Model file for the job. Use its own axes, mm. A direction names the side the tool comes from. Round coordinates to 2 decimals unless told otherwise and drop trailing zeros. Loops run counter-clockwise (first coordinate to the right, second up) from the corner with the lowest first, then second, coordinate; pieces in that order, holes last.
from build123d import *

# Parameters (mm, degrees)
BOSS_EXTRUDE1_DEPTH = 6


with BuildPart() as part:
    # Sketch1 → Boss-Extrude1 (new body)
    with BuildSketch(Plane.XY):
        Polygon((24.866162055, -35.317756725), (12.866162055, -35.317756725), (12.866162055, -26.332846246), (-17.133837945, -26.332846246), (-17.133837945, -35.317756725), (-29.133837945, -35.317756725), (-29.133837945, -53.317756725), (-17.133837945, -53.317756725), (-17.133837945, -59.317756725), (12.866162055, -59.317756725), (12.866162055, -53.317756725), (24.866162055, -53.317756725), align=None)
        Polygon((-7.133837945, -42.067756725), (-2.133837945, -49.067756725), (2.866162055, -42.067756725), align=None, mode=Mode.SUBTRACT)
    extrude(amount=BOSS_EXTRUDE1_DEPTH)


solid = part.part
Q1. Pull direction X, two halves, no side cores. Call faces 4 (the face through (-4.67, -45.52, 2.96)), 5 (the face through (0.33, -45.62, 2.96)), 6 (the face through (12.866, -56, 3)), 7 (the face through (19, -35.318, 3)): pulls with the +X half, pulls with the -X half, needs draft (parallel to the pull), parting line crosses it, or undercut.
Q2. Probe line 1 (Y direction, x = 13, z = 5.05); line 2 (X direction, y = -27.5, z = 5.1); line 3 (Y direction, x = -1, z = 0.85). List the from-to ranges inside material, lowest first.
Q3. Slice it at C-C on y = -44. Give the cut face in (x, z).
Q4. Tool access for faces 1 (the face through (12.866, -31, 3)), 2 (the face through (19, -53.318, 3)), 3 (the face through (-17.134, -31, 3)): list every direction of +Z, -Z, +X, -X, +Y, -Y with a clear straight run to the whole face (end or side of a thin tool).
Q5. Slice it at A-A on x = -5. Give the cut face in (y, z), plus the area to 3 significant figures.
Q6. Flat gauge pin, fed straight in: P1, Ø1.8, axis at y = -33, z = 2.5, coming from the +X side. Where does the tip first touch, or does it go through?
Q7. Slice it at D-D on x = 21.5. Give the cut face in (y, z).
Q8. Slice it at B-B on z = 2.95. Give the cut face in (x, y).
Reply:
1. face 4: undercut
1. face 5: undercut
1. face 6: pulls with the +X half
1. face 7: needs draft
2. line 1: y = -53.32 to -35.32
2. line 2: x = -17.13 to 12.87
2. line 3: y = -59.32 to -47.48, -42.07 to -26.33
3. outline: (-29.13, 0) - (-5.75, 0) - (-5.75, 6) - (-29.13, 6) - close; (1.49, 0) - (24.87, 0) - (24.87, 6) - (1.49, 6) - close
4. face 1: +Z, -Z, +X, +Y
4. face 2: +Z, -Z, +X, -Y
4. face 3: +Z, -Z, -X, +Y
5. outline: (-59.32, 0) - (-45.06, 0) - (-45.06, 6) - (-59.32, 6) - close; (-42.07, 0) - (-26.33, 0) - (-26.33, 6) - (-42.07, 6) - close
5. area: 180 mm2
6. P1: stops at x = 12.87
7. outline: (-53.32, 0) - (-35.32, 0) - (-35.32, 6) - (-53.32, 6) - close
8. outline: (-29.13, -53.32) - (-17.13, -53.32) - (-17.13, -59.32) - (12.87, -59.32) - (12.87, -53.32) - (24.87, -53.32) - (24.87, -35.32) - (12.87, -35.32) - (12.87, -26.33) - (-17.13, -26.33) - (-17.13, -35.32) - (-29.13, -35.32) - close; hole (-7.13, -42.07) - (-2.13, -49.07) - (2.87, -42.07) - close
